Work out the finished part from the listing and answer in its coordinate system (mm). Face numbers are marked on the shaded views. Coordinates: 2 decimals unless noted, no trailing zeros. Order: outer loops, then holes, each group sorted by start corner. A loop starts at its lowest first (then second) coordinate and runs counter-clockwise, first axis right, second up. Notation, with made-up numbers: M -17,71.5 L 9,71.5 A15 cw 9,79.5 Z; hole C -36.75,-35 d10. An arc over 180 degrees is marked long. Answer in a Markdown table with one row per item. Add a question column.
Item 1: The part is cut by section B-B (z = 247.65). Write down the section's boundary in (x, y) (3 decimals).
Item 2: The part is cut by section C-C (z = 109). Write down the section's boundary in (x, y) (3 decimals), then the cut area to 3 significant figures.
Item 3: Consider line 1 (X direction, y = 30, z = 143.5) (3 decimals); line 2 (X direction, y = 1.9, z = 247.65); line 3 (Y direction, x = 8, z = 69.5) (3 decimals). Determine where each line is inside the solid, lowest interval first. Write a range as from..to.
Item 4: The part is cut by section A-A (y = 16). Write down the section's boundary in (x, z) (3 decimals).
Item 5: The mould has two halves that part along X. Classify the marked faces 1, 2 and 3: released by +X, released by -X, zero draft, split by the parting line, or undercut.
Item 6: The part is cut by section D-D (x = 9.5). Write down the section's boundary in (y, z) (3 decimals), then the cut area to 3 significant figures.
Item 7: Flat-ended cylindrical pins translate along their axes: pin 1 Ø3.5 at (x, y) = (18, 24) entering from +Z; pin 2 Ø1.6 at (x, y) = (17, 25.5) entering from -Z. Find the tip coordinate at first contact, or state that the pin passes through.
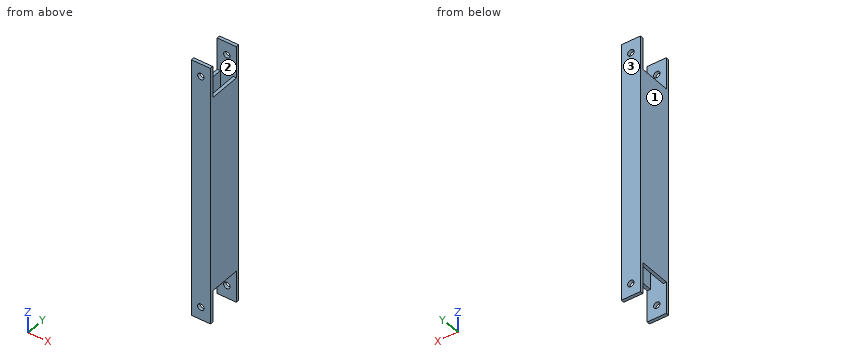
from build123d import *

# Parameters (mm, degrees)
SKETCH1_W           = 19.05
SKETCH1_H           = 38.1
SKETCH1_W_2         = 12.7
SKETCH1_H_2         = 31.75
BOSS_EXTRUDE1_DEPTH = 260.35
SKETCH2_W           = 19.05
SKETCH2_H           = 31.75
CUT_EXTRUDE1_DEPTH  = 31.75
SKETCH3_R           = 3.175
CUT_EXTRUDE2_DEPTH  = 264.811741589


with BuildPart() as part:
    # Sketch1 → Boss-Extrude1 (new body)
    with BuildSketch(Plane.XY):
        with Locations((9.525, 19.05)):
            Rectangle(SKETCH1_W, SKETCH1_H)
        with Locations((9.525, 19.05)):
            Rectangle(SKETCH1_W_2, SKETCH1_H_2, mode=Mode.SUBTRACT)
    extrude(amount=BOSS_EXTRUDE1_DEPTH)

    # Sketch2 → Cut-Extrude1 (cut)
    with BuildSketch(Plane.XY.offset(260.35)):
        with Locations((9.525, 19.05)):
            Rectangle(SKETCH2_W, SKETCH2_H)
    cut_extrude1 = extrude(amount=-CUT_EXTRUDE1_DEPTH, mode=Mode.SUBTRACT)

    # Sketch3 → Cut-Extrude2 (cut, through all)
    with BuildSketch(Plane(origin=(0, 38.1, 0), x_dir=(1, 0, 0), z_dir=(0, 1, 0))):
        with Locations(Location((9.525, -247.65, 0), (0, 0, 180))):
            Circle(SKETCH3_R)
    cut_extrude2 = extrude(amount=-CUT_EXTRUDE2_DEPTH, mode=Mode.SUBTRACT)

    # Mirror1: Cut-Extrude1, Cut-Extrude2 across plane
    add(cut_extrude1.mirror(Plane.XY.offset(130.175)), mode=Mode.SUBTRACT)
    add(cut_extrude2.mirror(Plane.XY.offset(130.175)), mode=Mode.SUBTRACT)


solid = part.part
Reply:
| question | item | result |
|---|---|---|
| 1 | outline | M 0,0 L 6.35,0 L 6.35,3.175 L 0,3.175 Z; M 0,34.925 L 6.35,34.925 L 6.35,38.1 L 0,38.1 Z; M 12.7,0 L 19.05,0 L 19.05,3.175 L 12.7,3.175 Z; M 12.7,34.925 L 19.05,34.925 L 19.05,38.1 L 12.7,38.1 Z |
| 2 | outline | M 0,0 L 19.05,0 L 19.05,38.1 L 0,38.1 Z; hole M 3.175,3.175 L 15.875,3.175 L 15.875,34.925 L 3.175,34.925 Z |
| 2 | area | 323 mm2 |
| 3 | line 1 | x = 0..3.175, 15.875..19.05 |
| 3 | line 2 | x = 0..6.35, 12.7..19.05 |
| 3 | line 3 | y = 0..3.175, 34.925..38.1 |
| 4 | outline | M 0,31.75 L 3.175,31.75 L 3.175,228.6 L 0,228.6 Z; M 15.875,31.75 L 19.05,31.75 L 19.05,228.6 L 15.875,228.6 Z |
| 5 | face 1 | released by -X |
| 5 | face 2 | undercut |
| 5 | face 3 | zero draft |
| 6 | outline | M 0,0 L 3.175,0 L 3.175,9.525 L 0,9.525 Z; M 0,15.875 L 3.175,15.875 L 3.175,244.475 L 0,244.475 Z; M 0,250.825 L 3.175,250.825 L 3.175,260.35 L 0,260.35 Z; M 34.925,0 L 38.1,0 L 38.1,9.525 L 34.925,9.525 Z; M 34.925,15.875 L 38.1,15.875 L 38.1,244.475 L 34.925,244.475 Z; M 34.925,250.825 L 38.1,250.825 L 38.1,260.35 L 34.925,260.35 Z |
| 6 | area | 1,570 mm2 |
| 7 | pin 1 | stops at z = 228.6 |
| 7 | pin 2 | stops at z = 31.75 |
